Read the model definition and answer for the solid it produces. Units are mm, in the model's axes. A direction names the side the tool comes from. Coordinates: 2 decimals unless noted, no trailing zeros. Loops run counter-clockwise (first coordinate to the right, second up) from the corner with the lowest first, then second, coordinate; pieces in that order, holes last. Notation, with made-up numbers: (-38.75, 18) -> (-15.75, 18) arc R35 ccw to (-15.75, 54) -> close; hole circle Ø4 at (22.25, 86). An arc over 180 degrees is marked (long way). Answer in a Markdown table with one row per item.
```python
from build123d import *

# Parameters (mm, degrees)
BOSS_EXTRUDE1_DEPTH = 4.699
SKETCH2_R           = 1.3335
BOSS_EXTRUDE2_DEPTH = 6.985


with BuildPart() as part:
    # Sketch1 → Boss-Extrude1 (new body)
    with BuildSketch(Plane(origin=(0, 0, 0), x_dir=(1, 0, 0), z_dir=(0, 1, 0))):
        Polygon((2.712968915, 0), (1.356484457, 2.3495), (-1.356484457, 2.3495), (-2.712968915, 0), (-1.356484457, -2.3495), (1.356484457, -2.3495), align=None)
    extrude(amount=BOSS_EXTRUDE1_DEPTH)

    # Sketch2 → Boss-Extrude2 (add)
    with BuildSketch(Plane.XZ):
        with Locations(Location((0, 0, 0), (0, 0, 90))):
            Circle(SKETCH2_R)
    extrude(amount=BOSS_EXTRUDE2_DEPTH)

    # Sketch5 → Cut-Revolve1 (revolve, cut)
    with BuildSketch(Plane(origin=(0, 0, 0), x_dir=(0, 0, -1), z_dir=(1, 0, 0))):
        Polygon((2.3495, 4.699), (3.223173217, 3.825326783), (3.223173217, 4.699), align=None)
    cut_revolve1 = revolve(axis=Axis((0, 4.699, 0), (0, 1, 0)), mode=Mode.SUBTRACT)

    # Mirror1: Cut-Revolve1 across plane
    add(cut_revolve1.mirror(Plane.ZX.offset(2.3495)), mode=Mode.SUBTRACT)


solid = part.part
```
1. A cutting plane is placed at A-A on y = 3.5. Give the vertices of the cut face in (x, z), and give its area (3 significant figures).
A:
| item | result |
|---|---|
| outline | (-2.71, 0) -> (-1.36, -2.35) -> (1.36, -2.35) -> (2.71, 0) -> (1.36, 2.35) -> (-1.36, 2.35) -> close |
| area | 19.1 mm2 |
2. A tool of negligible diameter and unlimited length cuts with its end or side. For faces 1 (the flat face through (0, 2, 2.35)), 2 (the cylindrical face through (0.81, -3.44, -1.06)), from which of +Z, -Z, +X, -X, +Y, -Y can it reach the whole face along a straight path? Write none if from no direction.
A:
| item | result |
|---|---|
| face 1 | +Z, +X, -X, +Y, -Y |
| face 2 | -Y |
3. Find the intervals of material crossed by probe 1 along Y at (x, z) = (1.3, -0.9); probe 2 along X at (y, z) = (4.25, -1.7); probe 3 along X at (y, z) = (-2, -0.7) (3 decimals), in increasing order.
A:
| item | result |
|---|---|
| probe 1 | y = 0 to 4.7 |
| probe 2 | x = -1.73 to 1.73 |
| probe 3 | x = -1.135 to 1.135 |
4. The mould has two halves that part along Y. Classify faces 3 (the flat face through (-2.025, 2.317, -1.191)), 4 (the conical face through (-1.244, 4.57, 2.143)), 5 (the conical face through (-1.23, 0.13, -2.15)): pulls with the +Y half, pulls with the -Y half, needs draft (parallel to the pull), parting line crosses it, or undercut.
A:
| item | result |
|---|---|
| face 3 | needs draft |
| face 4 | pulls with the +Y half |
| face 5 | pulls with the -Y half |
5. A cutting plane is placed at B-B on y = -5. Give the vertices of the cut face in (x, z).
A:
| item | result |
|---|---|
| outline | circle Ø2.67 at (0, 0) |
6. Given pin 1 Ø1 at (x, z) = (-2, -0.5) entering from -Y, flat-ended and moving along its own axis, determine where the tip first touches the part or whether it passes through.
A:
| item | result |
|---|---|
| pin 1 | stops at y = 0 |
